Autodesk Inventor part; units mm, degrees
ref_plane "YZ Plane" through (0, 0, 0) normal (1, 0, 0) x (0, 1, 0)
ref_plane "XZ Plane" through (0, 0, 0) normal (0, 1, 0) x (-1, 0, 0)
ref_plane "XY Plane" through (0, 0, 0) normal (0, 0, 1) x (1, 0, 0)
sketch "Boceto2" plane through (0, 0, 0) normal (1, 0, 0) x (0, 1, 0)
  line L0 (8, 5.1) -> (8, 0)
  line L1 (8, 0) -> (8, -5.1)
  line L2 (8, -5.1) -> (9.9, -5.1)
  line L3 (9.9, -5.1) -> (12, -3)
  line L4 (12, -3) -> (12, 3)
  line L5 (12, 3) -> (9.9, 5.1)
  line L6 (9.9, 5.1) -> (8, 5.1)
  line L7 (0, 19.536) -> (0, -22.6626)
  point P0 (0, 0)
  dimension "d2" = 6
  dimension "d3" = 5.1
  dimension "d4" = 4
  dimension "d5" = 135
  dimension "d6" = 5.1
  dimension "d7" = 8
revolve "Revolución1" add sketch "Boceto2" angle 360 about axis through (0, 0, 19.536) along (0, 0, -1)
properties part number "Rueda v" material "Caucho"
Read the model definition and answer for the solid it produces. Units are mm, in the model's axes. Give positions to 0.01 mm unless a question says otherwise; leave off trailing zeros. Loops run counter-clockwise (first coordinate to the right, second up) from the corner with the lowest first, then second, coordinate; pieces in that order, holes last.
Item 1: The part is cut by section C-C (z = -3.75). Write down the section's boundary in (x, y).
Item 2: The part is cut by section D-D (z = 1.5). Write down the section's boundary in (x, y), and give its area (3 significant figures).
Item 3: Each of these flat-tipped pins is pushed along its axis until it touches: pin 1 Ø5 at (x, z) = (-6.5, -0.5) entering from +Y; pin 2 Ø1 at (y, z) = (7, 2.5) entering from +X; pin 3 Ø6 at (y, z) = (9.5, 0.5) entering from -X. Where does it stop, or does it pass through?
Item 4: The part is cut by section A-A (y = 0). Write down the section's boundary in (x, z), and give its area (3 significant figures).
Item 5: Find the intervals of material crossed by line 1 along X through (y, z) = (0, 1); line 2 along X through (y, z) = (-2, 2.75); line 3 along Y through (x, z) = (-3.25, 0.75), in increasing order.
Item 6: The mould has two halves that part along X. Classify faces 1 (the conical face through (3.01, 9.57, 4.97)), 2 (the flat face through (-7.3, -3.7, -5.1)), 3 (the cylindrical face through (-7.81, -1.73, -0.07)): released by +X, released by -X, zero draft, split by the parting line, or undercut.
Taken from the geometry:
1. outline: circle Ø22.5 at (0, 0); hole circle Ø16 at (0, 0)
2. outline: circle Ø24 at (0, 0); hole circle Ø16 at (0, 0)
2. area: 251 mm2
3. pin 1: stops at y = 11.31
3. pin 2: stops at x = 10.09
3. pin 3: stops at x = -10.09
4. outline: (-12, -3) - (-9.9, -5.1) - (-8, -5.1) - (-8, 5.1) - (-9.9, 5.1) - (-12, 3) - close; (8, -5.1) - (9.9, -5.1) - (12, -3) - (12, 3) - (9.9, 5.1) - (8, 5.1) - close
4. area: 72.8 mm2
5. line 1: x = -12 to -8, 8 to 12
5. line 2: x = -11.83 to -7.75, 7.75 to 11.83
5. line 3: y = -11.55 to -7.31, 7.31 to 11.55
6. face 1: split by the parting line
6. face 2: zero draft
6. face 3: undercut
